Check sheet for the modelled part. Datum: model origin and axes. Units: mm. A direction names the side the tool comes from. Round coordinates to 2 decimals unless told otherwise and drop trailing zeros. Order: outer loops, then holes, each group sorted by start corner. A loop starts at its lowest first (then second) coordinate and runs counter-clockwise, first axis right, second up. Notation, with made-up numbers: (27.5, 56) -> (69.5, 56) arc R29 cw to (69.5, 83) -> close; hole circle Ø8 at (-34.75, 0). An arc over 180 degrees is marked (long way). Answer in a Markdown table with one row per item. Add a question column.
1. Depth check by flat-ended pin: P1, Ø5.5, axis at x = -22.5, z = -0.5, coming from the -Y side; P2, Ø4.5, axis at y = 3, z = -3.5, coming from the -X side. Enter the tip coordinate at first touch or a pass-through.
2. Sectioned sample at A-A, the plane x = -34. Record the boundary of the cut face in (y, z), then the cut area to 3 significant figures.
3. Access from +Z, -Z, +X, -X, +Y, -Y to the whole of each face (thin tool, end or side, straight path). Record for faces 4 (the flat face through (0, -10, -5)), 5 (the flat face through (-26, 0, 0)), 6 (the flat face through (-20, -8, 0)).
4. Sectioned sample at D-D, the plane y = 3. Record the boundary of the cut face in (x, z).
5. Sectioned sample at C-C, the plane y = -16.5. Record the boundary of the cut face in (x, z), then the cut area to 3 significant figures.
6. Sectioned sample at B-B, the plane z = 0. Record the boundary of the cut face in (x, y).
7. Material ranges on L1, parallel to X at y = -14, z = 0; L2, parallel to X at y = -10, z = 0; L3, parallel to X at y = -15, z = 8.5, recorded low to high. Write a range as from..to.
8. Draft check along X on faces 1 (the cylindrical face through (-25.453, -14.902, 0.716)), 2 (the cylindrical face through (7.6, 8.97, 4.67)), 3 (the flat face through (15, 0, 0)). Enter one of: +X half, -X half, draft (parallel to the pull), parting line (faces both ways), or undercut.
```python
from build123d import *

# Parameters (mm, degrees)
BLOCK_SKETCH_W          = 40
BLOCK_SKETCH_H          = 44
BLOCK_DEPTH             = 22
NECK_SKETCH_W           = 15
NECK_SKETCH_H           = 10.1125
REGULATOR_PORT_SKETCH_W = 15
REGULATOR_PORT_SKETCH_H = 7.2
SIDE_PORT_Y_SKETCH_W    = 5.5
SIDE_PORT_Y_SKETCH_H    = 15


with BuildPart() as part:
    # Block Sketch → Block (new, symmetric)
    with BuildSketch(Plane.XY):
        with Locations((-20, 0)):
            Rectangle(BLOCK_SKETCH_W, BLOCK_SKETCH_H)
    extrude(amount=BLOCK_DEPTH, both=True)

    # Neck Sketch → Neck (revolve)
    with BuildSketch(Plane.XY, mode=Mode.PRIVATE) as neck_sk:
        with Locations((7.5, 5.05625)):
            Rectangle(NECK_SKETCH_W, NECK_SKETCH_H)
    revolve(neck_sk.sketch.rotate(Axis((-1000, 0, 0), (1, 0, 0)), 90), axis=Axis((-1000, 0, 0), (1, 0, 0)))

    # Regulator Port Sketch → Regulator Port (revolve, cut)
    with BuildSketch(Plane.XY, mode=Mode.PRIVATE) as regulator_port_sk:
        with Locations((-33.5, 3.6)):
            Rectangle(REGULATOR_PORT_SKETCH_W, REGULATOR_PORT_SKETCH_H)
    revolve(regulator_port_sk.sketch.rotate(Axis((-1000, 0, 0), (1, 0, 0)), 90), axis=Axis((-1000, 0, 0), (1, 0, 0)), mode=Mode.SUBTRACT)

    # Side Port -Y Sketch → Side Port -Y (revolve, cut)
    with BuildSketch(Plane.XY, mode=Mode.PRIVATE) as side_port_y_sk:
        with Locations((-17.25, -15.5)):
            Rectangle(SIDE_PORT_Y_SKETCH_W, SIDE_PORT_Y_SKETCH_H)
    revolve(side_port_y_sk.sketch.rotate(Axis((-20, -40, 0), (0, 1, 0)), 90), axis=Axis((-20, -40, 0), (0, 1, 0)), mode=Mode.SUBTRACT)


solid = part.part
```
Answer key:
| question | item | result |
|---|---|---|
| 1 | P1 | stops at y = -8 |
| 1 | P2 | stops at x = -26 |
| 2 | outline | (-22, -22) -> (22, -22) -> (22, 22) -> (-22, 22) -> close; hole circle Ø14.4 at (0, 0) |
| 2 | area | 1,770 mm² |
| 3 | face 4 | +X |
| 3 | face 5 | -X |
| 3 | face 6 | -Y |
| 4 | outline | (-40, -22) -> (0, -22) -> (0, -9.66) -> (15, -9.66) -> (15, 9.66) -> (0, 9.66) -> (0, 22) -> (-40, 22) -> (-40, 6.55) -> (-26, 6.55) -> (-26, -6.55) -> (-40, -6.55) -> close |
| 5 | outline | (-40, -22) -> (0, -22) -> (0, 22) -> (-40, 22) -> close; hole circle Ø11 at (-20, 0) |
| 5 | area | 1,660 mm² |
| 6 | outline | (-40, -22) -> (-25.5, -22) -> (-25.5, -8) -> (-14.5, -8) -> (-14.5, -22) -> (0, -22) -> (0, -10.11) -> (15, -10.11) -> (15, 10.11) -> (0, 10.11) -> (0, 22) -> (-40, 22) -> (-40, 7.2) -> (-26, 7.2) -> (-26, -7.2) -> (-40, -7.2) -> close |
| 7 | L1 | x = -40..-25.5, -14.5..0 |
| 7 | L2 | x = -40..-25.5, -14.5..15 |
| 7 | L3 | x = -40..0 |
| 8 | face 1 | undercut |
| 8 | face 2 | draft |
| 8 | face 3 | +X half |
